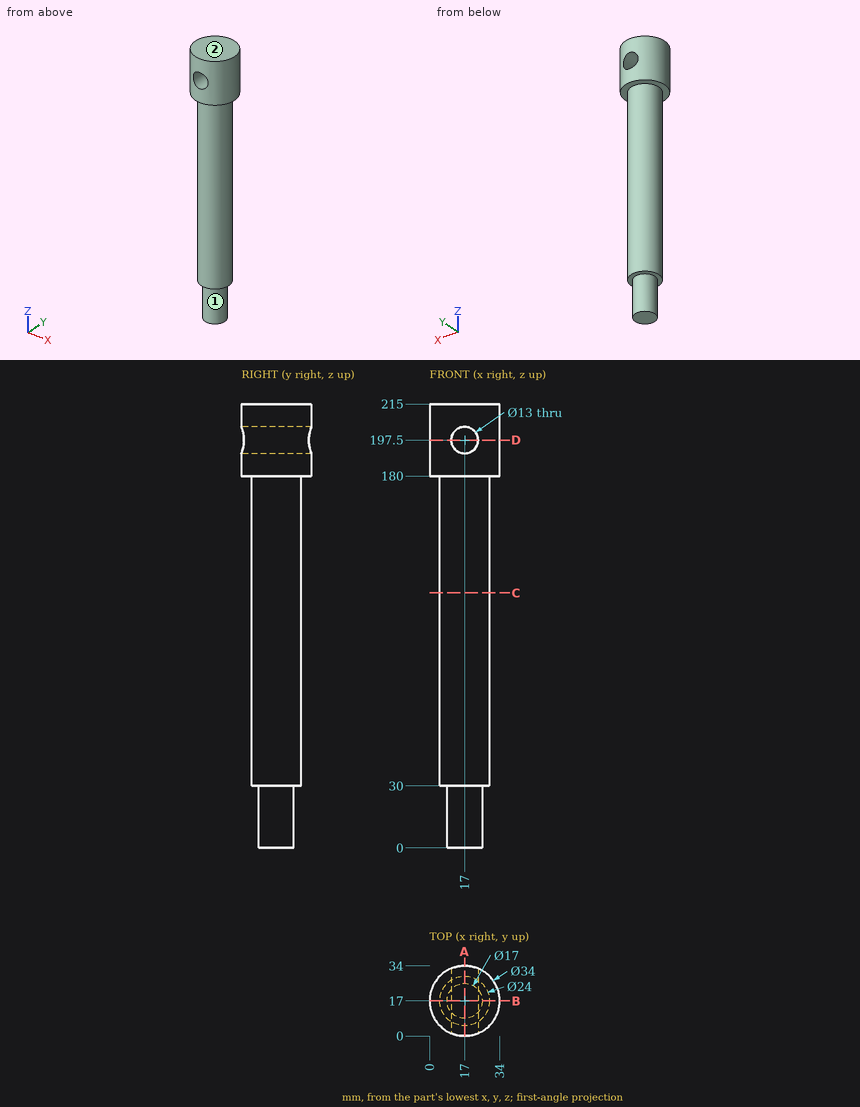
Here's the drawing with two shaded views (mm, measured from the low corner). I have some questions. A direction names the side the tool comes from. Round coordinates to 2 decimals unless told otherwise and drop trailing zeros. Write each loop counter-clockwise with the first axis right and the second up, starting at its lowest first coordinate (ties: lowest second). Pieces come first, ordered by that corner, then holes. Notation, with made-up numbers: M 52,-5 L 92,-5 A13 cw 92,17 Z; hole C 63.5,27 d6. An arc over 180 degrees is marked long. Answer in a Markdown table with one row per item. Add a question column.
Q1. Imagine slicing it at B-B (y = 17). Please give me the cut outline in (x, z).
Q2. Will these pins go through, and if not, where does the flat tip stop? pin 1 Ø10 at (y, z) = (6.5, 102) entering from +X; pin 2 Ø1 at (x, y) = (23.5, 9) entering from -Z; pin 3 Ø5 at (x, z) = (9.5, 123.5) entering from -Y.
Q3. If I drill on line 1 (Z direction, x = 17, y = 9); line 2 (X direction, y = 17.5, z = 197.5); line 3 (X direction, y = 16, z = 128), over which ranges is the centre line in solid material (lowest first)? Write a range as from..to.
Q4. Imagine slicing it at A-A (x = 17). Please give me the cut outline in (y, z), then the cut area to 3 significant figures.
Q5. Imagine slicing it at C-C (z = 123.5). Please give me the cut outline in (x, y), then the cut area to 3 significant figures.
Q6. Imagine slicing it at D-D (z = 197.5). Please give me the cut outline in (x, y), then the cut area to 3 significant figures.
Q7. On a 3-axis mill with a long thin cutter (end or side, diameter ignored), from which of +Z, -Z, +X, -X, +Y, -Y can I reach the whole of each face in a straight line? I mean the marked faces 1 and 2. Say none if no direction works.
Values:
| question | item | result |
|---|---|---|
| 1 | outline | M 0,180 L 5,180 L 5,30 L 8.5,30 L 8.5,0 L 25.5,0 L 25.5,30 L 29,30 L 29,180 L 34,180 L 34,215 L 0,215 Z; hole C 17,197.5 d13 |
| 2 | pin 1 | x = 27.67 |
| 2 | pin 2 | z = 30 |
| 2 | pin 3 | y = 6.09 |
| 3 | line 1 | 0..191, 204..215 |
| 3 | line 2 | 0.01..10.5, 23.5..33.99 |
| 3 | line 3 | 5.04..28.96 |
| 4 | outline | M 0,180 L 5,180 L 5,30 L 8.5,30 L 8.5,0 L 25.5,0 L 25.5,30 L 29,30 L 29,180 L 34,180 L 34,191 L 0,191 Z; M 0,204 L 34,204 L 34,215 L 0,215 Z |
| 4 | area | 4,860 mm^2 |
| 5 | outline | C 17,17 d24 |
| 5 | area | 452 mm^2 |
| 6 | outline | M 10.5,1.29 L 10.5,32.71 A17 ccw Z; M 23.5,1.29 A17 ccw 23.5,32.71 Z |
| 6 | area | 477 mm^2 |
| 7 | face 1 | -Z |
| 7 | face 2 | +Z, +X, -X, +Y, -Y |
